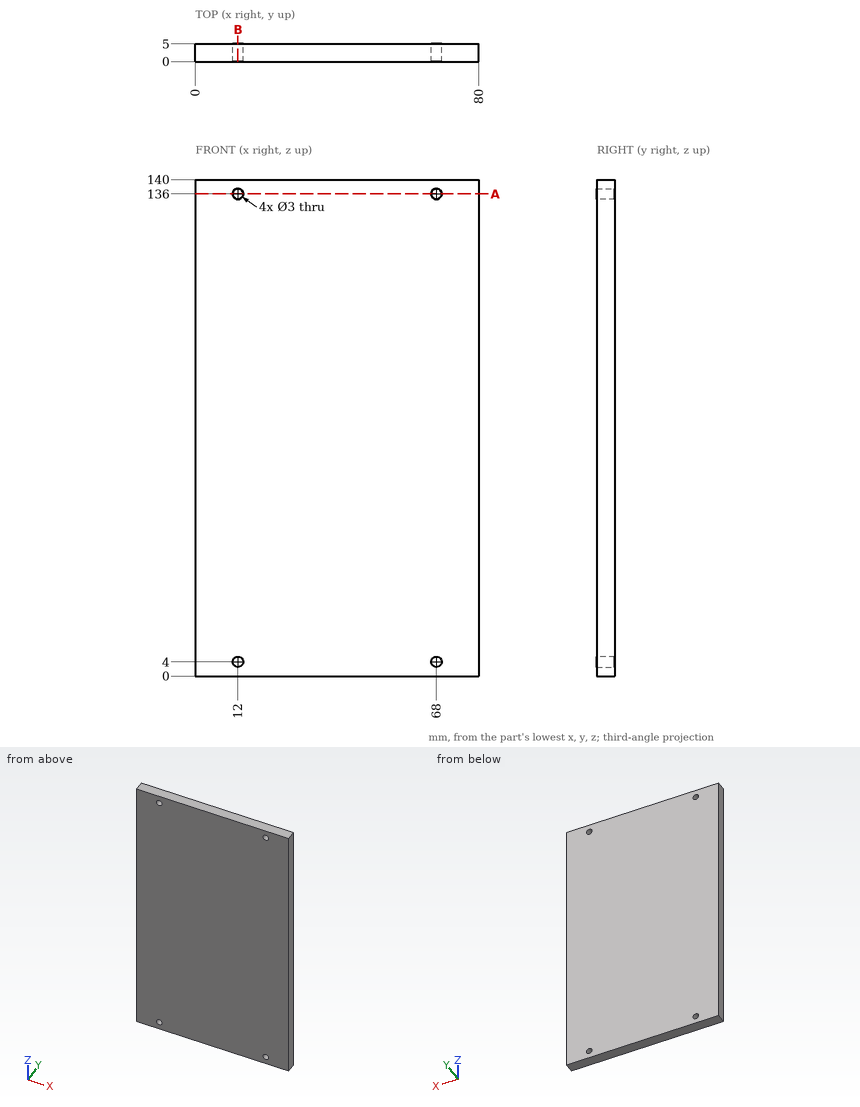
Source: three-view drawing plus pictorial views. Frame: mm from the lowest corner of the part. Give positions to 0.01 mm unless a question says otherwise; leave off trailing zeros. Write each loop counter-clockwise with the first axis right and the second up, starting at its lowest first coordinate (ties: lowest second). Pieces come first, ordered by that corner, then holes. Notation, with made-up numbers: (-29, 1) - (16, 1) arc R18 ccw to (16, 14) - close; hole circle Ø9 at (47, 87.25). An arc over 180 degrees is marked (long way). Write item = value, one per line. Start each with the question number.
Q1. Cut plane B-B, the plane x = 12. Return loops of the section in (y, z), then the cut area to 3 significant figures.
Q2. Cut plane A-A, the plane z = 136. Return loops of the section in (x, y), then the cut area to 3 significant figures.
Q3. Material intervals for probe 1 along Z at (x, y) = (12, 4.05); probe 2 along X at (y, z) = (2.2, 136); probe 3 along Z at (x, y) = (11.5, 3.3), sorted ascending.
Computed values:
q1.outline = (0, 0) - (5, 0) - (5, 2.5) - (0, 2.5) - close; (0, 5.5) - (5, 5.5) - (5, 134.5) - (0, 134.5) - close; (0, 137.5) - (5, 137.5) - (5, 140) - (0, 140) - close
q1.area = 670 mm²
q2.outline = (0, 0) - (10.5, 0) - (10.5, 5) - (0, 5) - close; (13.5, 0) - (66.5, 0) - (66.5, 5) - (13.5, 5) - close; (69.5, 0) - (80, 0) - (80, 5) - (69.5, 5) - close
q2.area = 370 mm²
q3.probe_1 = 0 to 2.5, 5.5 to 134.5, 137.5 to 140
q3.probe_2 = 0 to 10.5, 13.5 to 66.5, 69.5 to 80
q3.probe_3 = 0 to 2.59, 5.41 to 134.59, 137.41 to 140
